from build123d import *

# Parameters (mm, degrees)
BOSS_EXTRUDE1_DEPTH = 80
SKETCH2_R           = 50
BOSS_EXTRUDE2_DEPTH = 10
SKETCH3_R           = 47.09331112
CUT_EXTRUDE1_DEPTH  = 10
SKETCH4_R           = 50
BOSS_EXTRUDE3_DEPTH = 25
SKETCH5_R           = 47.09331112
CUT_EXTRUDE2_DEPTH  = 20


with BuildPart() as part:
    # Sketch1 → Boss-Extrude1 (new body)
    with BuildSketch(Plane(origin=(0, 0, 0), x_dir=(0, 0, -1), z_dir=(1, 0, 0))):
        Polygon((40.609756098, 22.658536585), (40.609756098, 78.658536585), (-4.390243902, 78.658536585), (-4.390243902, -51.341463415), (5.609756098, -51.341463415), (5.609756098, 68.658536585), (30.609756098, 68.658536585), (30.609756098, 22.658536585), align=None)
    extrude(amount=BOSS_EXTRUDE1_DEPTH)

    # Sketch2 → Boss-Extrude2 (add)
    with BuildSketch(Plane(origin=(0, 30, 0), x_dir=(1, 0, 0), z_dir=(0, 1, 0))):
        with Locations((40.088163703, -47.932474998)):
            Circle(SKETCH2_R)
    extrude(amount=BOSS_EXTRUDE2_DEPTH)

    # Sketch3 → Cut-Extrude1 (cut)
    with BuildSketch(Plane(origin=(0, 40, 0), x_dir=(1, 0, 0), z_dir=(0, 1, 0))):
        with Locations(Location((40.088163703, -47.932474998, 0), (0, 0, 67.607335059))):
            Circle(SKETCH3_R)
    extrude(amount=-CUT_EXTRUDE1_DEPTH, mode=Mode.SUBTRACT)

    # Sketch4 → Boss-Extrude3 (add)
    with BuildSketch(Plane(origin=(0, -51, 0), x_dir=(1, 0, 0), z_dir=(0, 1, 0))):
        with Locations((40.088163703, -47.932474998)):
            Circle(SKETCH4_R)
    extrude(amount=BOSS_EXTRUDE3_DEPTH)

    # Sketch5 → Cut-Extrude2 (cut)
    with BuildSketch(Plane(origin=(0, -26, 0), x_dir=(1, 0, 0), z_dir=(0, 1, 0))):
        with Locations(Location((40.088163703, -47.932474998, 0), (0, 0, 67.607335059))):
            Circle(SKETCH5_R)
    extrude(amount=-CUT_EXTRUDE2_DEPTH, mode=Mode.SUBTRACT)


solid = part.part
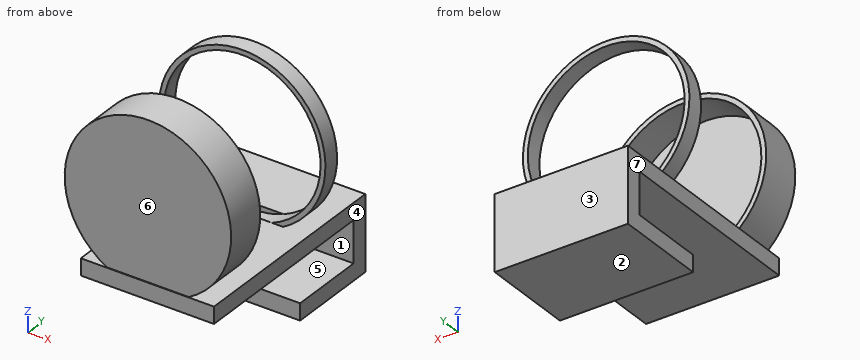
Can you work these out from the model? Positions are in its coordinate system, mm. Face numbers are marked on the shaded views. A direction names the side the tool comes from. Give positions to 0.01 mm unless a question says otherwise; leave off trailing zeros. Loops run counter-clockwise (first coordinate to the right, second up) from the corner with the lowest first, then second, coordinate; pieces in that order, holes last. Notation, with made-up numbers: (89, -8) - (133, -8) arc R19 cw to (133, 13) - close; hole circle Ø9 at (-12, 0). An arc over 180 degrees is marked (long way). Answer as a JSON object with one key per item and string values.
Q1. Imagine slicing it at A-A on y = 66.5. Write out the boundary of the cut face in (x, z), plus the area to 3 significant figures.
Geometry says:
{"outline": "(0, -40.61) - (80, -40.61) - (80, -30.61) - (0, -30.61) - close; (0, -5.61) - (80, -5.61) - (80, 4.39) - (0, 4.39) - close", "area": "1,600 mm²"}
Q2. Imagine slicing it at B-B on z = 45.5. Write out the boundary of the cut face in (x, y).
Geometry says:
{"outline": "(-9.85, -51) - (90.03, -51) - (90.03, -26) - (87.12, -26) - (87.12, -46) - (-6.94, -46) - (-6.94, -26) - (-9.85, -26) - close; (-9.85, 30) - (-6.94, 30) - (-6.94, 40) - (-9.85, 40) - close; (87.12, 30) - (90.03, 30) - (90.03, 40) - (87.12, 40) - close"}
Q3. Imagine slicing it at C-C on x = 41. Write out the boundary of the cut face in (y, z), plus the area to 3 significant figures.
Geometry says:
{"outline": "(-51.34, -5.61) - (68.66, -5.61) - (68.66, -30.61) - (22.66, -30.61) - (22.66, -40.61) - (78.66, -40.61) - (78.66, 4.39) - (40, 4.39) - (40, 0.85) - (30, 0.85) - (30, 4.39) - (-26, 4.39) - (-26, 0.85) - (-46, 0.85) - (-46, 95.02) - (-26, 95.02) - (-26, 97.92) - (-51, 97.92) - (-51, 4.39) - (-51.34, 4.39) - close; (30, 95.02) - (40, 95.02) - (40, 97.92) - (30, 97.92) - close", "area": "2,560 mm²"}
Q4. If I drill on L1, parallel to Z at x = 51.5, y = 41.5; L2, parallel to Z at x = 56, y = 35; L3, parallel to Z at x = 51, y = -39, over which ranges is the centre line in solid material (lowest first)?
Geometry says:
{"L1": "-40.61 to -30.61, -5.61 to 4.39", "L2": "-40.61 to -30.61, -5.61 to 3.61, 92.26 to 95.33", "L3": "-5.61 to 2.12, 93.74 to 96.73"}
Q5. Which directions (+Z, -Z, +X, -X, +Y, -Y) give clear straight access to the entire face, cutting with the end or side of a thin tool? Please do the marked faces 4, 5, 6 and 7.
Geometry says:
{"face 4": "-Z, +X, +Y, -Y", "face 5": "+X, -X, -Y", "face 6": "+Z, +X, -X, -Y", "face 7": "-Z, -X, +Y, -Y"}
Q6. Imagine slicing it at D-D on x = 2. Write out the boundary of the cut face in (y, z), plus the area to 3 significant figures.
Geometry says:
{"outline": "(-51.34, -5.61) - (68.66, -5.61) - (68.66, -30.61) - (22.66, -30.61) - (22.66, -40.61) - (78.66, -40.61) - (78.66, 4.39) - (-51.34, 4.39) - close; (-51, 15.54) - (-26, 15.54) - (-26, 20.24) - (-46, 20.24) - (-46, 75.63) - (-26, 75.63) - (-26, 80.33) - (-51, 80.33) - close; (30, 15.54) - (40, 15.54) - (40, 20.24) - (30, 20.24) - close; (30, 75.63) - (40, 75.63) - (40, 80.33) - (30, 80.33) - close", "area": "2,720 mm²"}
Q7. Will these pins go through, and if not, where does the flat tip stop? P1, Ø12.5, axis at x = 35.5, z = -20.5, coming from the -Y side; P2, Ø11, axis at x = 49.5, z = -33, coming from the -Y side; P3, Ø5, axis at y = 38, z = 58.5, coming from the +X side.
Geometry says:
{"P1": "y = 68.66", "P2": "y = 22.66", "P3": "x = 89.43"}
Q8. If we mould it in two halves opening along Z, with no side actions, what happens to the marked faces 1, 2 and 3? For each: pulls with the +Z half, pulls with the -Z half, needs draft (parallel to the pull), parting line crosses it, or undercut.
Geometry says:
{"face 1": "undercut", "face 2": "pulls with the -Z half", "face 3": "needs draft"}
